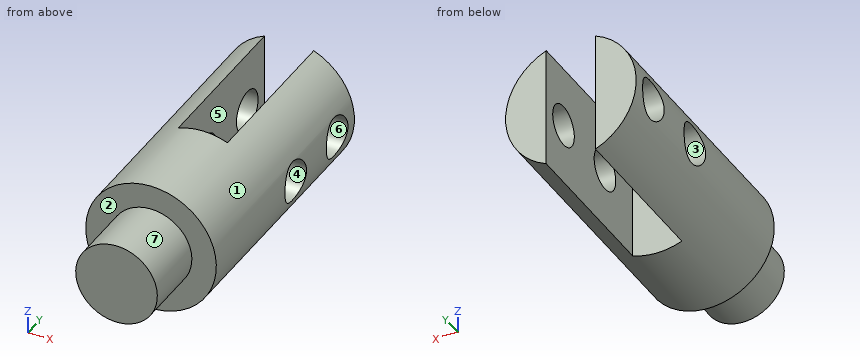
from build123d import *

# Parameters (mm, degrees)
SKETCH3_W          = 9.5758
SKETCH3_H          = 52.44541986
CUT_EXTRUDE2_DEPTH = 31.75
SKETCH4_R          = 3.97256
SKETCH4_R_2        = 3.96875
CUT_EXTRUDE3_DEPTH = 26.4


with BuildPart() as part:
    # Sketch1 → Revolve1 (revolve)
    with BuildSketch(Plane(origin=(0, 0, 0), x_dir=(0, 0, -1), z_dir=(1, 0, 0))):
        Polygon((0, 0), (-12.7, 0), (-12.7, -50.8), (-7.9375, -50.8), (-7.9375, -63.5), (0, -63.5), (0, -50.8), align=None)
    revolve(axis=Axis((0, 54.105122951, 0), (0, -1, 0)))

    # Sketch3 → Cut-Extrude2 (cut)
    with BuildSketch(Plane(origin=(0, 0, 0), x_dir=(1, 0, 0), z_dir=(0, 1, 0))):
        Rectangle(SKETCH3_W, SKETCH3_H)
    extrude(amount=-CUT_EXTRUDE2_DEPTH, mode=Mode.SUBTRACT)

    # Sketch4 → Cut-Extrude3 (cut, through all)
    with BuildSketch(Plane(origin=(12.7, 0, 0), x_dir=(0, 0, -1), z_dir=(1, 0, 0))):
        with Locations((0, -6.35)):
            Circle(SKETCH4_R)
        with Locations((0, -21.59)):
            Circle(SKETCH4_R_2)
    extrude(amount=-CUT_EXTRUDE3_DEPTH, mode=Mode.SUBTRACT)


solid = part.part
Input: part model. Units: mm. Frame: model coordinates. Face numbers are marked on the shaded views. A direction names the side the tool comes from. Coordinates: 2 decimals unless noted, no trailing zeros. Order: outer loops, then holes, each group sorted by start corner. A loop starts at its lowest first (then second) coordinate and runs counter-clockwise, first axis right, second up. Notation, with made-up numbers: M 71.25,61 L 81.25,61 A22 cw 81.25,76 Z; hole C 26.5,61 d2. An arc over 180 degrees is marked long. Write item = value, one per line. Start each with the question number.
(1) Pull-direction query (Z, two-part tool) for the marked faces 1, 2, 3 and 4; classes: released by +Z, released by -Z, zero draft, split by the parting line, or undercut.
(2) Reachability of the marked faces 5, 6 and 7 from +Z, -Z, +X, -X, +Y, -Y: full face, straight path, thin tool, end or side. Return the list, or none.
(3) Section C-C on z = 0. Output: boundary loops of the cut face in (x, y).
(4) Line query: line 1 along Y through (x, z) = (10.5, 0); line 2 along Y through (x, z) = (-10.5, -1.5); line 3 along Y through (x, z) = (-9, 8.75). Output: solid intervals per line, ascending. Write a range as [from, to].
(5) Section A-A on y = -21.59. Output: boundary loops of the cut face in (x, z).
(6) Section D-D on x = -10.25. Output: boundary loops of the cut face in (y, z).
(7) First-contact query: P1, Ø2, axis at x = -8.5, z = -4, coming from the -Y side; P2, Ø7, axis at y = -17, z = -4.5, coming from the -X side; P3, Ø5, axis at x = 3.5, y = -46, coming from the +Z side. Flat tips, straight axial feed; report the tip coordinate or a pass-through.
(8) Section B-B on x = 0. Output: boundary loops of the cut face in (y, z), and give its area (3 significant figures).
Result set:
q1.face_1 = split by the parting line
q1.face_2 = zero draft
q1.face_3 = undercut
q1.face_4 = undercut
q2.face_5 = +Z, -Z, +Y
q2.face_6 = +X, -X
q2.face_7 = -Y
q3.outline = M -12.7,-50.8 L -7.94,-50.8 L -7.94,-63.5 L 7.94,-63.5 L 7.94,-50.8 L 12.7,-50.8 L 12.7,-25.56 L 4.79,-25.56 L 4.79,-31.75 L -4.79,-31.75 L -4.79,-25.56 L -12.7,-25.56 Z; M -12.7,-17.62 L -4.79,-17.62 L -4.79,-10.32 L -12.7,-10.32 Z; M -12.7,-2.38 L -4.79,-2.38 L -4.79,0 L -12.7,0 Z; M 4.79,-17.62 L 12.7,-17.62 L 12.7,-10.32 L 4.79,-10.32 Z; M 4.79,-2.38 L 12.7,-2.38 L 12.7,0 L 4.79,0 Z
q4.line_1 = [-50.8, -25.56], [-17.62, -10.32], [-2.38, 0]
q4.line_2 = [-50.8, -25.26], [-17.92, -10.03], [-2.67, 0]
q4.line_3 = [-50.8, 0]
q5.outline = M -12.06,-3.97 A12.7 ccw -4.79,-11.76 L -4.79,-3.97 Z; M -12.06,3.97 L -4.79,3.97 L -4.79,11.76 A12.7 ccw Z; M 4.79,-11.76 A12.7 ccw 12.06,-3.97 L 4.79,-3.97 Z; M 4.79,3.97 L 12.06,3.97 A12.7 ccw 4.79,11.76 Z
q6.outline = M -50.8,-7.5 L 0,-7.5 L 0,7.5 L -50.8,7.5 Z; hole C -21.59,0 d7.94; hole C -6.35,0 d7.95
q7.P1 = -50.8
q7.P2 = -12.66
q7.P3 = 12.66
q8.outline = M -63.5,-7.94 L -50.8,-7.94 L -50.8,-12.7 L -31.75,-12.7 L -31.75,12.7 L -50.8,12.7 L -50.8,7.94 L -63.5,7.94 Z
q8.area = 685 mm²
